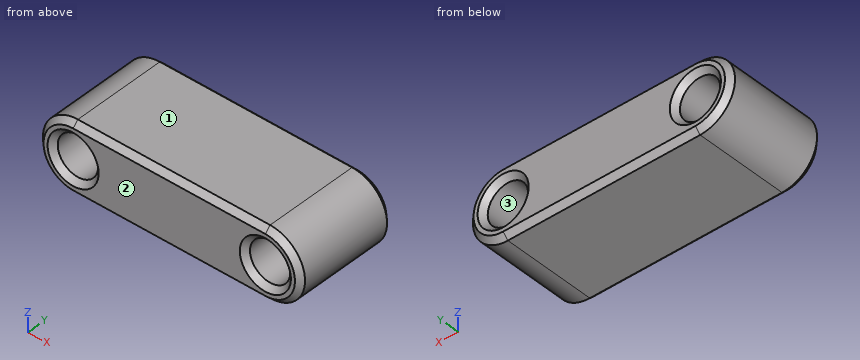
```python
from build123d import *

# Parameters (mm, degrees)
SKETCH1_R           = 1.5
BOSS_EXTRUDE1_DEPTH = 3.85
CHAMFER2_SIZE       = 0.4


with BuildPart() as part:
    # Sketch1 → Boss-Extrude1 (new body, symmetric)
    with BuildSketch(Plane(origin=(0, 0, 0), x_dir=(1, 0, 0), z_dir=(0, 1, 0))):
        with BuildLine():
            Line((-5.963610114, 2.6), (8.336389886, 2.6))
            ThreePointArc((8.336389886, 2.6), (10.936389886, 0), (8.336389886, -2.6))
            Line((8.336389886, -2.6), (-5.963610114, -2.6))
            ThreePointArc((-5.963610114, -2.6), (-8.563610114, 0), (-5.963610114, 2.6))
        make_face()
        with Locations((-5.963610114, 0)):
            Circle(SKETCH1_R, mode=Mode.SUBTRACT)
        with Locations((8.336389886, 0)):
            Circle(SKETCH1_R, mode=Mode.SUBTRACT)
    extrude(amount=BOSS_EXTRUDE1_DEPTH, both=True)

    # Chamfer2
    chamfer2_edges = [part.edges().sort_by_distance(p)[0] for p in [
        (-7.463610114, -3.85, 0),
        (-7.463610114, 3.85, 0),
        (10.936389886, 3.85, 0),
        (6.836389886, -3.85, 0),
        (6.836389886, 3.85, 0),
        (1.186389886, 3.85, -2.6),
        (-8.563610114, 3.85, 0),
        (1.186389886, -3.85, -2.6),
        (10.936389886, -3.85, 0),
        (1.186389886, -3.85, 2.6),
        (-8.563610114, -3.85, 0),
        (1.186389886, 3.85, 2.6),
    ]]
    chamfer(chamfer2_edges, length=CHAMFER2_SIZE)


solid = part.part
```
For this review, take the finished solid that the model builds, in its own axes (mm). Face numbers are marked on the shaded views. Coordinates: 2 decimals unless noted, no trailing zeros. Write each loop counter-clockwise with the first axis right and the second up, starting at its lowest first coordinate (ties: lowest second). Pieces come first, ordered by that corner, then holes. Notation, with made-up numbers: (-7, 54.25) - (12, 54.25) arc R23 cw to (12, 75.25) - close; hole circle Ø5 at (56.25, -10.5). An arc over 180 degrees is marked (long way). Answer in a Markdown table with one row per item. Add a question column.
Q1. For P1, Ø1, axis at y = -0.5, z = -0.5, coming from the -X side; P2, Ø3, axis at y = 0.5, z = -2, coming from the +X side, all flat-tipped, find the tip position at first contact; note any pin that passes through.
Q2. We need section C-C, the plane z = -1.3. Count the separate pieces of the cut face and the enclosed holes in it, and give its area (3 significant figures).
Q3. Draft analysis for pull direction Z (two halves, no side actions). For the marked faces 1, 2 and 3, state which applies: +Z half, -Z half, draft (parallel to the pull), parting line (faces both ways), or undercut.
Q4. For probe 1 along X at (y, z) = (-0.25, 0); probe 2 along X at (y, z) = (0, -0.45); probe 3 along Z at (x, y) = (-6.5, 2.5), list the stretches that pass through material, from the lowest coordinate up.
Q5. We need section A-A, the plane z = 0. State the section outline as (x, y) points.
Q6. We need section B-B, the plane y = -1. State the section outline as (x, z) points.
Answer list:
| question | item | result |
|---|---|---|
| 1 | P1 | stops at x = -8.56 |
| 1 | P2 | stops at x = 10.89 |
| 2 | separate pieces | 3 |
| 2 | enclosed holes | 0 |
| 2 | area | 120 mm2 |
| 3 | face 1 | +Z half |
| 3 | face 2 | draft |
| 3 | face 3 | undercut |
| 4 | probe 1 | x = -8.56 to -7.46, -4.46 to 6.84, 9.84 to 10.94 |
| 4 | probe 2 | x = -8.52 to -7.39, -4.53 to 6.91, 9.77 to 10.9 |
| 4 | probe 3 | z = -2.54 to -1.4, 1.4 to 2.54 |
| 5 | outline | (-8.56, -3.45) - (-8.16, -3.85) - (-7.86, -3.85) - (-7.46, -3.45) - (-7.46, 3.45) - (-7.86, 3.85) - (-8.16, 3.85) - (-8.56, 3.45) - close; (-4.46, -3.45) - (-4.06, -3.85) - (6.44, -3.85) - (6.84, -3.45) - (6.84, 3.45) - (6.44, 3.85) - (-4.06, 3.85) - (-4.46, 3.45) - close; (9.84, -3.45) - (10.24, -3.85) - (10.54, -3.85) - (10.94, -3.45) - (10.94, 3.45) - (10.54, 3.85) - (10.24, 3.85) - (9.84, 3.45) - close |
| 6 | outline | (-5.96, -2.6) - (8.34, -2.6) arc R2.6 ccw to (8.34, 2.6) - (-5.96, 2.6) arc R2.6 ccw to start; hole circle Ø3 at (-5.96, 0); hole circle Ø3 at (8.34, 0) |
